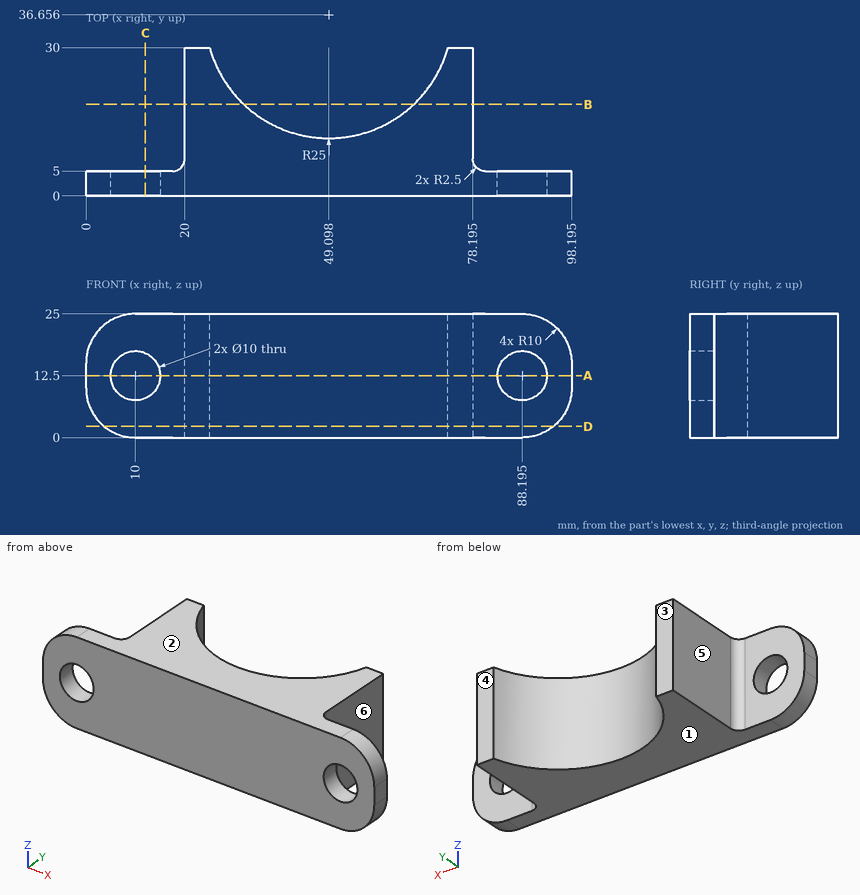
For this review, use the dimensioned drawing (mm, ordinates from the lowest corner) and the shaded views. A direction names the side the tool comes from. Round coordinates to 2 decimals unless told otherwise and drop trailing zeros. Order: outer loops, then holes, each group sorted by start corner. A loop starts at its lowest first (then second) coordinate and runs counter-clockwise, first axis right, second up. Notation, with made-up numbers: (54, 79) -> (79, 79) arc R36 ccw to (79, 118) -> close; hole circle Ø6 at (86.5, -13.75). An arc over 180 degrees is marked (long way). Use CSV: the item, a comma, the result in double quotes. Start each with the question number.
(1) Insertion check: pin 1 (7 mm diameter, centred on y = 19, z = 15.5, fed in from +X) (1 decimal); pin 2 (8 mm diameter, centred on x = 88.2, z = 12.5, fed in from +Y); pin 3 (4 mm diameter, centred on y = 24, z = 3.5, fed in from -X); pin 4 (9 mm diameter, centred on x = 85.5, z = 18, fed in from +Y). Each pin has a flat end and moves straight along its axis. Give the tip position at first contact, or say it passes through.
(2) Mouldability with a two-part tool opening along Z and no side actions: class the marked faces 1, 2 and 3 as pulls with the +Z half, pulls with the -Z half, needs draft (parallel to the pull), parting line crosses it, or undercut.
(3) Consider section D-D on z = 2.25. Write out the cut boundary in (x, y) (1 decimal).
(4) Wall thickness on probe 1 along Z at (x, y) = (10, 1.3); probe 2 along Y at (x, z) = (92, 18.75); probe 3 along X at (y, z) = (4, 9.75) (1 decimal): over which ranges is each line inside the solid? List them lowest first. Write a range as from..to.
(5) Consider section C-C on x = 12. Write out the cut boundary in (y, z).
(6) Consider section A-A on z = 12.5. Write out the cut boundary in (x, y) (1 decimal), and give its area (3 significant figures).
(7) Tool access review of the marked faces 4, 5 and 6: name each direction out of +Z, -Z, +X, -X, +Y, -Y from which nothing blocks a thin tool from reaching the whole face with its end or side.
(8) Consider section B-B on y = 18.5. Write out the cut boundary in (x, z) (1 decimal).
Responses:
1,pin 1,"x = 78.2"
1,pin 2,"through"
1,pin 3,"x = 20"
1,pin 4,"y = 5"
2,face 1,"pulls with the -Z half"
2,face 2,"pulls with the +Z half"
2,face 3,"needs draft"
3,outline,"(3.7, 0) -> (94.5, 0) -> (94.5, 5) -> (80.7, 5) arc R2.5 cw to (78.2, 7.5) -> (78.2, 30) -> (73.2, 30) arc R25 cw to (25, 30) -> (20, 30) -> (20, 7.5) arc R2.5 cw to (17.5, 5) -> (3.7, 5) -> close"
4,probe 1,"0..7.5, 17.5..25"
4,probe 2,"0..5"
4,probe 3,"0..5.8, 14.2..84, 92.4..98.2"
5,outline,"(0, 0) -> (5, 0) -> (5, 7.92) -> (0, 7.92) -> close; (0, 17.08) -> (5, 17.08) -> (5, 25) -> (0, 25) -> close"
6,outline,"(0, 0) -> (5, 0) -> (5, 5) -> (0, 5) -> close; (15, 0) -> (83.2, 0) -> (83.2, 5) -> (80.7, 5) arc R2.5 cw to (78.2, 7.5) -> (78.2, 30) -> (73.2, 30) arc R25 cw to (25, 30) -> (20, 30) -> (20, 7.5) arc R2.5 cw to (17.5, 5) -> (15, 5) -> close; (93.2, 0) -> (98.2, 0) -> (98.2, 5) -> (93.2, 5) -> close"
6,area,"1,200 mm²"
7,face 4,"+Z, -Z, +X, -X, +Y"
7,face 5,"+Z, -Z, -X, +Y"
7,face 6,"+Z, -Z, +X, +Y"
8,outline,"(20, 0) -> (31.9, 0) -> (31.9, 25) -> (20, 25) -> close; (66.3, 0) -> (78.2, 0) -> (78.2, 25) -> (66.3, 25) -> close"
